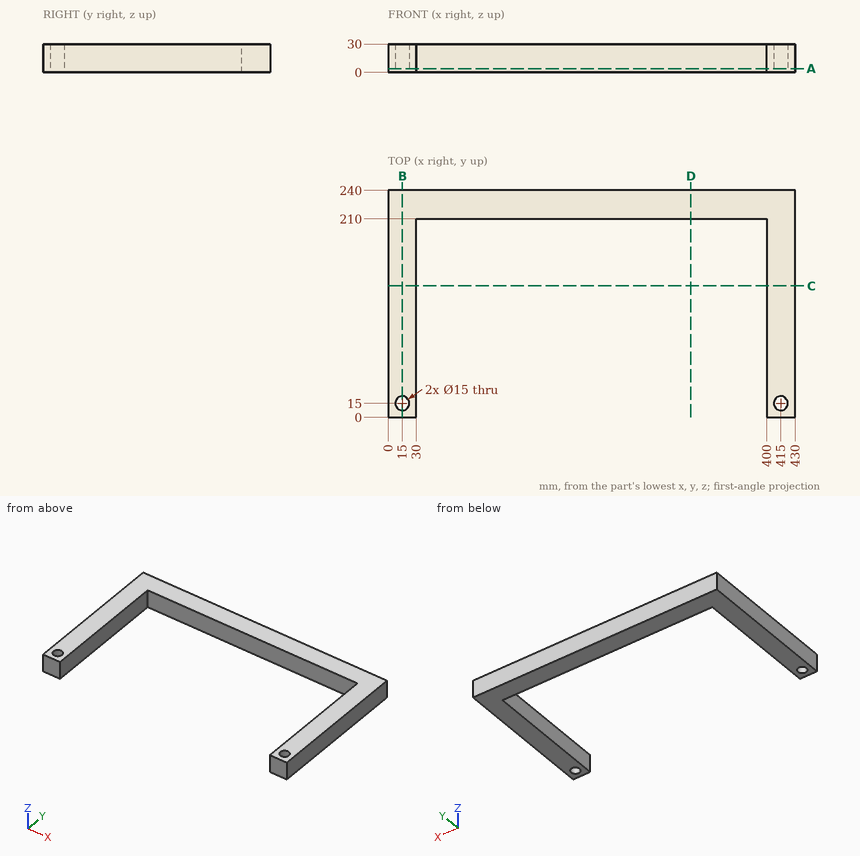
Part print with two shaded views. Sizes in mm from the minimum x, y, z corner. Round coordinates to 2 decimals unless told otherwise and drop trailing zeros. Write each loop counter-clockwise with the first axis right and the second up, starting at its lowest first coordinate (ties: lowest second). Pieces come first, ordered by that corner, then holes. Notation, with made-up numbers: (50, 46) - (64, 46) arc R11 cw to (64, 51) - close; hole circle Ø5 at (-28, 3). An arc over 180 degrees is marked (long way). Answer as CSV lines item,"result".
Q1. Cut at C-C (y = 139). Write the cut outline in (x, z).
Report:
outline,"(0, 0) - (30, 0) - (30, 30) - (0, 30) - close; (400, 0) - (430, 0) - (430, 30) - (400, 30) - close"
Q2. Drill centre lines: probe 1 along Y at (x, z) = (15, 17); probe 2 along X at (y, z) = (181, 19); probe 3 along Y at (x, z) = (163.5, 23.5). Where is each one in solid material? Low to high. Write a range as [from, to].
Report:
probe 1,"y = [0, 7.5], [22.5, 240]"
probe 2,"x = [0, 30], [400, 430]"
probe 3,"y = [210, 240]"
Q3. Drop flat-ended pins along their axis: pin 1 (19.5 mm diameter, centred on x = 415, y = 15, fed in from -Z); pin 2 (9 mm diameter, centred on x = 15, y = 15, fed in from -Z); pin 3 (1.5 mm diameter, centred on x = 182, z = 15.5, fed in from -Y). Give the stop position or say it passes through.
Report:
pin 1,"stops at z = 0"
pin 2,"passes through"
pin 3,"stops at y = 210"
Q4. Cut at D-D (x = 320). Write the cut outline in (y, z).
Report:
outline,"(210, 0) - (240, 0) - (240, 30) - (210, 30) - close"
Q5. Cut at A-A (z = 4). Write the cut outline in (x, y), and give its area (3 significant figures).
Report:
outline,"(0, 0) - (30, 0) - (30, 210) - (400, 210) - (400, 0) - (430, 0) - (430, 240) - (0, 240) - close; hole circle Ø15 at (15, 15); hole circle Ø15 at (415, 15)"
area,"25,100 mm^2"
Q6. Cut at B-B (x = 15). Write the cut outline in (y, z).
Report:
outline,"(0, 0) - (7.5, 0) - (7.5, 30) - (0, 30) - close; (22.5, 0) - (240, 0) - (240, 30) - (22.5, 30) - close"
